For this review, take the finished solid that the model builds, in its own axes (mm). Coordinates: 2 decimals unless noted, no trailing zeros. Loops run counter-clockwise (first coordinate to the right, second up) from the corner with the lowest first, then second, coordinate; pieces in that order, holes last. Notation, with made-up numbers: (32, -20) - (78, -20) arc R33 ccw to (78, 11) - close; hole circle Ø3 at (-18.5, 53). An arc over 180 degrees is marked (long way). One line per item, written item: value. Start each with the question number.
1. Take a section at C-C, the plane z = 5.25. State the section outline as (x, y) points, and give its area (3 significant figures).
2. Insertion check: pin 1 (4 mm diameter, centred on x = 0, y = 20.5, fed in from -Z); pin 2 (1.9 mm diameter, centred on x = 0, y = -20.5, fed in from -Z). Each pin has a flat end and moves straight along its axis. Give the tip position at first contact, or say it passes through.
3. To check wall thickness, follow line 1 (Y direction, x = 0, z = 5); line 2 (Y direction, x = 1, z = 5.5). State the ranges of each line that lie inside material, in increasing order. Write a range as from..to.
4. The part is to be moulded in two halves that separate along Y. For faces 1 (the face through (0, 0, 7)), 2 (the face through (0, -24.5, 4)), 3 (the face through (-0.208, 22.086, 3.648)), say which applies: released by +Y, released by -Y, zero draft, split by the parting line, or undercut.
5. Take a section at B-B, the plane y = 20.5. State the section outline as (x, z) points.
6. Take a section at A-A, the plane x = 0. State the section outline as (y, z) points.
```python
from build123d import *

# Parameters (mm, degrees)
F0_W    = 16
F0_H    = 49
F0_R    = 1.6
F3_SIZE = 0.2


with BuildPart() as f2:
    # F2: sweep along a path in F1
    with BuildLine(Plane.XZ) as f2_path:
        Line((0, 0), (0, 7))
    # F0 (on Top) → F2 (sweep)
    with BuildSketch(Plane.XY):
        Rectangle(F0_W, F0_H)
        with Locations((0, -20.5)):
            Circle(F0_R, mode=Mode.SUBTRACT)
        with Locations((0, 20.5)):
            Circle(F0_R, mode=Mode.SUBTRACT)
    sweep(path=f2_path.line)

    # F3
    f3_edges = [f2.edges().sort_by_distance(p)[0] for p in [
        (8, 0, 0),
        (0, -24.5, 0),
        (0, 24.5, 0),
        (-8, 0, 0),
        (-1.6, -20.5, 0),
        (-1.6, 20.5, 0),
    ]]
    chamfer(f3_edges, length=F3_SIZE)


solid = f2.part
```
Solutions:
1. outline: (-8, -24.5) - (8, -24.5) - (8, 24.5) - (-8, 24.5) - close; hole circle Ø3.2 at (0, -20.5); hole circle Ø3.2 at (0, 20.5)
1. area: 768 mm2
2. pin 1: z = 0
2. pin 2: through
3. line 1: -24.5..-22.1, -18.9..18.9, 22.1..24.5
3. line 2: -24.5..-21.75, -19.25..19.25, 21.75..24.5
4. face 1: zero draft
4. face 2: released by -Y
4. face 3: undercut
5. outline: (-8, 0.2) - (-7.8, 0) - (-1.8, 0) - (-1.6, 0.2) - (-1.6, 7) - (-8, 7) - close; (1.6, 0.2) - (1.8, 0) - (7.8, 0) - (8, 0.2) - (8, 7) - (1.6, 7) - close
6. outline: (-24.5, 0.2) - (-24.3, 0) - (-22.3, 0) - (-22.1, 0.2) - (-22.1, 7) - (-24.5, 7) - close; (-18.9, 0.2) - (-18.7, 0) - (18.7, 0) - (18.9, 0.2) - (18.9, 7) - (-18.9, 7) - close; (22.1, 0.2) - (22.3, 0) - (24.3, 0) - (24.5, 0.2) - (24.5, 7) - (22.1, 7) - close
